Autodesk Inventor part; units mm, degrees
ref_plane "YZ Plane" through (0, 0, 0) normal (1, 0, 0) x (0, 1, 0)
ref_plane "XZ Plane" through (0, 0, 0) normal (0, 1, 0) x (-1, 0, 0)
ref_plane "XY Plane" through (0, 0, 0) normal (0, 0, 1) x (1, 0, 0)
sketch "Sketch1" plane through (0, 0, 0) normal (0, 1, 0) x (-1, 0, 0)
  line L0 (-26.95, 0) -> (26.95, 0)
  line L1 (-26.95, 0) -> (-85.687, 70)
  line L2 (85.687, 70) -> (26.95, 0)
  line L3 (90.6172, 13.6467) -> (45.6023, -40)
  line L4 (45.6023, -40) -> (-45.6023, -40)
  line L5 (-45.6023, -40) -> (-90.6172, 13.6467)
  line L6 (0, 0) -> (0, -40) construction
  arc A0 (90.6172, 13.6467) -> (85.687, 70) centre (59.9755, 39.3582) ccw
  arc A1 (-85.687, 70) -> (-90.6172, 13.6467) centre (-59.9755, 39.3582) ccw
  point P0 (0, 70)
  dimension "d1" = 53.9
  dimension "d3" = 40
  dimension "d5" = 40
  dimension "d16" = 130
  dimension "d17" = 70
extrude "Extrusion1" add sketch "Sketch1" along normal blind 15
sketch "Sketch2" plane through (0, 0, 0) normal (0, -1, 0) x (1, 0, 0)
  line L0 (-26.95, 0) -> (26.95, 0)
  line L1 (-85.687, 70) -> (-26.95, 0)
  line L2 (-45.6023, -40) -> (-90.6172, 13.6467) construction
  line L3 (45.6023, -40) -> (-45.6023, -40) construction
  line L4 (90.6172, 13.6467) -> (45.6023, -40) construction
  line L5 (26.95, 0) -> (85.687, 70)
  line L6 (-97.5632, 53.039) -> (-36.2762, -20)
  line L7 (-36.2762, -20) -> (36.2762, -20)
  line L8 (36.2762, -20) -> (97.5632, 53.039)
  line L9 (-85.687, 70) -> (-26.95, 0)
  line L10 (26.95, 0) -> (85.687, 70)
  arc A0 (-85.687, 70) -> (-90.6172, 13.6467) centre (-59.9755, 39.3582) ccw
  arc A1 (90.6172, 13.6467) -> (85.687, 70) centre (59.9755, 39.3582) ccw
  point P0 (0, 0)
  dimension "d8" = 20
  dimension "d9" = 20
  dimension "d10" = 20
extrude "Extrusion2" cut sketch "Sketch2" against normal blind 3
fillet "Fillet1" radius 10.7 4 edges at (-85.687, 9, 70) (85.687, 9, 70) (-45.6023, 7.5, -40) (45.6023, 7.5, -40)
equation "\"d5\" = d3"
equation "\"d16\" = Лоток_угол"
equation "\"d9\" = d8"
equation "\"d10\" = d8"
equation "\"BendRadius\" = Thickness"
equation "\"BendReliefWidth\" = Thickness"
equation "\"BendReliefDepth\" = 0.5 * Thickness"
equation "\"TransitionRadius\" = BendRadius"
equation "\"JacobiRadiusSize\" = BendRadius"
equation "\"GapSize\" = Thickness"
properties part number "ДМФ 033 держатель лотка"
Design review of the part built by this model. Coordinates are the model's own, in mm. A direction names the side the tool comes from. Round coordinates to 2 decimals unless told otherwise and drop trailing zeros. Write each loop counter-clockwise with the first axis right and the second up, starting at its lowest first coordinate (ties: lowest second). Pieces come first, ordered by that corner, then holes.
Item 1: For faces 1 (the cylindrical face through (-99.81, 7.4, 35.71)), 2 (the flat face through (0, 9, 0)), 3 (the flat face through (66.49, 1.48, 16.01)), list the 3-axis set-ups (+Z, -Z, +X, -X, +Y, -Y) from which the entire face can be reached by the end or side of a thin tool; tool diameter is ignored.
Item 2: We need section C-C on x = -4.5. Write out the cut boundary in (y, z).
Item 3: For probe 1 along Z at (x, y) = (32, 2.5); probe 2 along X at (y, z) = (10, 50) (3 decimals); probe 3 along X at (y, z) = (13.5, 23), list the stretches that pass through material, from the lowest coordinate up.
Item 4: Clearance check with flat-ended pins moving along their axes: pin 1 Ø3 at (x, z) = (-13.5, -11) entering from -Y; pin 2 Ø6 at (y, z) = (12.5, 25.5) entering from +X; pin 3 Ø0.9 at (x, y) = (8.5, 1.5) entering from +Z. State where each tip first meets the part, or that it passes through.
Item 5: We need section D-D on z = 55.5. Write out the cut boundary in (x, y).
Item 6: We need section A-A on z = 22. Write out the cut boundary in (x, y), and give its area (3 significant figures).
Item 7: We need section B-B on y = 9.5. Write out the cut boundary in (x, z), and give its area (3 significant figures).
Returned:
1. face 1: -X, +Y, -Y
1. face 2: +Z, +Y, -Y
1. face 3: +Z, -Y
2. outline: (0, -40) - (15, -40) - (15, 0) - (3, 0) - (3, -20) - (0, -20) - close
3. probe 1: z = -40 to -20
3. probe 2: x = -98.534 to -68.905, 68.905 to 98.534
3. probe 3: x = -96.48 to -46.25, 46.25 to 96.48
4. pin 1: stops at y = 3
4. pin 2: stops at x = 98.47
4. pin 3: stops at z = -20
5. outline: (-96.57, 3) - (-73.52, 3) - (-73.52, 15) - (-96.57, 15) - close; (73.52, 3) - (96.57, 3) - (96.57, 15) - (73.52, 15) - close
6. outline: (-96.01, 0) - (-71.52, 0) - (-71.52, 3) - (-45.41, 3) - (-45.41, 15) - (-96.01, 15) - close; (45.41, 3) - (71.52, 3) - (71.52, 0) - (96.01, 0) - (96.01, 15) - (45.41, 15) - close
6. area: 1,360 mm2
7. outline: (-95.1, 58.49) arc R40 ccw to (-90.62, 13.65) - (-48.81, -36.18) arc R10.7 ccw to (-40.61, -40) - (40.61, -40) arc R10.7 ccw to (48.81, -36.18) - (90.62, 13.65) arc R40 ccw to (95.1, 58.49) arc R10.7 ccw to (77.51, 60.25) - (26.95, 0) - (-26.95, 0) - (-77.51, 60.25) arc R10.7 ccw to start
7. area: 10,200 mm2
